```python
from build123d import *

# Parameters (mm, degrees)
SKETCH2_W           = 25.654
SKETCH2_H           = 6.604
BOSS_EXTRUDE1_DEPTH = 6.35


with BuildPart() as part:
    # Sketch2 → Boss-Extrude1 (new body)
    with BuildSketch(Plane(origin=(0, 0, 0), x_dir=(1, 0, 0), z_dir=(0, 0, -1))):
        Polygon((-82.55, 73.64), (-82.55, 0), (-82.55, -6.35), (-101.6, -6.35), (-101.6, 0), (-101.6, 31.75), (-155.575, 31.75), (-155.575, 0), (-171.45, 0), (-171.45, -6.35), (-196.85, -6.35), (-196.85, 0), (-196.85, 73.64), (-196.85, 86.34), (-171.45, 86.34), (-171.45, 73.64), (-107.95, 73.64), (-107.95, 86.34), (-82.55, 86.34), align=None)
        with Locations((-139.7, 55.895)):
            Rectangle(SKETCH2_W, SKETCH2_H, mode=Mode.SUBTRACT)
    extrude(amount=BOSS_EXTRUDE1_DEPTH)


solid = part.part
```
Design review of the part built by this model. Coordinates are the model's own, in mm. A direction names the side the tool comes from. Coordinates: 2 decimals unless noted, no trailing zeros. Write each loop counter-clockwise with the first axis right and the second up, starting at its lowest first coordinate (ties: lowest second). Pieces come first, ordered by that corner, then holes. Notation, with made-up numbers: M 71,41.25 L 108,41.25 A16 cw 108,68.25 Z; hole C 73.5,-28.5 d10. An arc over 180 degrees is marked long. Answer as a JSON object with one key per item and string values.
Item 1: Wall thickness on probe 1 along Y at (x, z) = (-135, -3); probe 2 along X at (y, z) = (-15.5, -5.5) (3 decimals); probe 3 along X at (y, z) = (-80, -5.25): over which ranges is each line inside the solid? List them lowest first.
Outcome:
{"probe 1": "-73.64 to -59.2, -52.59 to -31.75", "probe 2": "-196.85 to -155.575, -101.6 to -82.55", "probe 3": "-196.85 to -171.45, -107.95 to -82.55"}
Item 2: Add section B-B, the plane z = -3.75. Give the boundary of the cut face in (x, y) (3 decimals), and give its area (3 significant figures).
Outcome:
{"outline": "M -196.85,-86.34 L -171.45,-86.34 L -171.45,-73.64 L -107.95,-73.64 L -107.95,-86.34 L -82.55,-86.34 L -82.55,6.35 L -101.6,6.35 L -101.6,-31.75 L -155.575,-31.75 L -155.575,0 L -171.45,0 L -171.45,6.35 L -196.85,6.35 Z; hole M -152.527,-59.197 L -126.873,-59.197 L -126.873,-52.593 L -152.527,-52.593 Z", "area": "7,460 mm²"}
Item 3: Draft analysis for pull direction X (two halves, no side actions). For faces 1 (the flat face through (-196.85, -41, -3)), 2 (the flat face through (-152.527, -56, -3)), 3 (the flat face through (-95, -86.34, -3)), state which applies: pulls with the +X half, pulls with the -X half, needs draft (parallel to the pull), parting line crosses it, or undercut.
Outcome:
{"face 1": "pulls with the -X half", "face 2": "undercut", "face 3": "needs draft"}
Item 4: Add section C-C, the plane x = -105.5. Give the boundary of the cut face in (y, z), and give its area (3 significant figures).
Outcome:
{"outline": "M -86.34,-6.35 L -31.75,-6.35 L -31.75,0 L -86.34,0 Z", "area": "347 mm²"}
Item 5: Add section D-D, the plane x = -162.5. Give the boundary of the cut face in (y, z), and give its area (3 significant figures).
Outcome:
{"outline": "M -73.64,-6.35 L 0,-6.35 L 0,0 L -73.64,0 Z", "area": "468 mm²"}
Item 6: Machinability: for faces 4 (the flat face through (-140, -73.64, -3)), 5 (the flat face through (-126.873, -56, -3)), 6 (the flat face through (-92, 6.35, -3)), 7 (the flat face through (-171.45, 3, -3)), which of the approach directions +Z, -Z, +X, -X, +Y, -Y give a long, thin tool a straight path to every point of the face, cutting with its end or side? Answer none if there is none.
Outcome:
{"face 4": "+Z, -Z, -Y", "face 5": "+Z, -Z", "face 6": "+Z, -Z, +X, -X, +Y", "face 7": "+Z, -Z, +Y"}
Item 7: Add section A-A, the plane y = -3.5. Give the boundary of the cut face in (x, z) (3 decimals), and give its area (3 significant figures).
Outcome:
{"outline": "M -196.85,-6.35 L -155.575,-6.35 L -155.575,0 L -196.85,0 Z; M -101.6,-6.35 L -82.55,-6.35 L -82.55,0 L -101.6,0 Z", "area": "383 mm²"}
